Work out the finished part from the listing and answer in its coordinate system (mm). Coordinates: 2 decimals unless noted, no trailing zeros. Loops run counter-clockwise (first coordinate to the right, second up) from the corner with the lowest first, then second, coordinate; pieces in that order, holes last. Notation, with made-up numbers: (71, 16.25) -> (93, 16.25) arc R13 cw to (93, 31.25) -> close; hole circle Ø4 at (42, 47). An arc over 180 degrees is marked (long way). Use a Markdown table: item, result.
from build123d import *

# Parameters (mm, degrees)
SKETCH1_W             = 450
SKETCH1_H             = 192
BOSS_EXTRUDE1_DEPTH   = 3
SKETCH2_R             = 30
CUT_EXTRUDE1_DEPTH    = 605.559191308
M10_CLEARANCE_SLOT1_D = 11


with BuildPart() as part:
    # Sketch1 → Boss-Extrude1 (new body)
    with BuildSketch(Plane.XY):
        with Locations((160.880387918, 36.737934288)):
            Rectangle(SKETCH1_W, SKETCH1_H)
    extrude(amount=BOSS_EXTRUDE1_DEPTH)

    # Sketch2 → Cut-Extrude1 (cut, through all)
    with BuildSketch(Plane(origin=(-44.574932583, -288.564846201, -49), x_dir=(-1, 0, 0), z_dir=(0, 0, -1))):
        with Locations(Location((-325.455320501, 287.298203547, 0), (0, 0, 90))):
            Circle(SKETCH2_R)
    extrude(amount=-CUT_EXTRUDE1_DEPTH, mode=Mode.SUBTRACT)

    # M10 Clearance Slot1 (through all)
    with Locations(Plane(origin=(-44.574932583, -288.564846201, -49), x_dir=(-1, 0, 0), z_dir=(0, 0, -1))):
        with Locations((-380.455320501, 390.298203547), (-205.455320501, 390.298203547), (-30.455320501, 390.298203547), (-30.455320501, 259.298203547), (-205.455320501, 259.298203547), (-380.455320501, 259.298203547)):
            Hole(M10_CLEARANCE_SLOT1_D / 2)


solid = part.part
Q1. Consider line 1 (X direction, y = 0, z = 0.7); line 2 (Y direction, x = -11.5, z = 1.65); line 3 (Y direction, x = 264, z = 0.9). Determine where each line is inside the solid, lowest interval first. Write a range as [from, to].
Solved:
| item | result |
|---|---|
| line 1 | [-64.12, 250.91], [310.85, 385.88] |
| line 2 | [-59.26, -34.1], [-24.43, 96.9], [106.57, 132.74] |
| line 3 | [-59.26, -26.07], [23.53, 132.74] |
Q2. Determine the mould class of faces 1 (the flat face through (158, 38, 0)), 2 (the cylindrical face through (-15.312, -34.636, 1.521)) for opening direction Y: pulls with the +Y half, pulls with the -Y half, needs draft (parallel to the pull), parting line crosses it, or undercut.
Solved:
| item | result |
|---|---|
| face 1 | needs draft |
| face 2 | undercut |
Q3. Section A-A on y = -10.5 is taken. Determine the outline of the cut face in (x, z).
Solved:
| item | result |
|---|---|
| outline | (-64.12, 0) -> (252.34, 0) -> (252.34, 3) -> (-64.12, 3) -> close; (309.42, 0) -> (385.88, 0) -> (385.88, 3) -> (309.42, 3) -> close |
Q4. Section B-B on z = 0.9 is taken. Determine the outline of the cut face in (x, y).
Solved:
| item | result |
|---|---|
| outline | (-64.12, -59.26) -> (385.88, -59.26) -> (385.88, 132.74) -> (-64.12, 132.74) -> close; hole circle Ø11 at (-14.12, -29.27); hole circle Ø11 at (-14.12, 101.73); hole circle Ø11 at (160.88, -29.27); hole circle Ø11 at (160.88, 101.73); hole circle Ø60 at (280.88, -1.27); hole circle Ø11 at (335.88, -29.27); hole circle Ø11 at (335.88, 101.73) |
Q5. Section C-C on y = 11.5 is taken. Determine the outline of the cut face in (x, z), and give its area (3 significant figures).
Solved:
| item | result |
|---|---|
| outline | (-64.12, 0) -> (253.73, 0) -> (253.73, 3) -> (-64.12, 3) -> close; (308.03, 0) -> (385.88, 0) -> (385.88, 3) -> (308.03, 3) -> close |
| area | 1,190 mm² |
